Work out the finished part from the listing and answer in its coordinate system (mm). Face numbers are marked on the shaded views. A direction names the side the tool comes from. Coordinates: 2 decimals unless noted, no trailing zeros. Order: outer loops, then holes, each group sorted by start corner. A loop starts at its lowest first (then second) coordinate and runs counter-clockwise, first axis right, second up. Notation, with made-up numbers: M 8.25,31.5 L 35.25,31.5 A12 cw 35.25,41.5 Z; hole C -20,65.5 d6. An arc over 180 degrees is marked long. Answer in a Markdown table with one row per item. Add a question column.
Item 1: Which of the six approach directions +Z, -Z, +X, -X, +Y, -Y give full straight-line access (tool end or side, diameter ignored) to the marked faces 1 and 2?
Item 2: Flat-ended cylindrical pins translate along their axes: pin 1 Ø0.9 at (x, z) = (-1, 0.5) entering from -Y; pin 2 Ø0.9 at (x, y) = (-1.5, 0.5) entering from -Z; pin 3 Ø0.7 at (x, z) = (-1, 0) entering from +Y. Find the tip coordinate at first contact, or state that the pin passes through.
Item 3: The mould has two halves that part along Y. Classify the marked faces 3, 4 and 5: released by +Y, released by -Y, zero draft, split by the parting line, or undercut.
Item 4: The part is cut by section B-B (z = 0). Write down the section's boundary in (x, y).
Item 5: Consider line 1 (X direction, y = -0.65, z = 0.2); line 2 (Y direction, x = -1, z = -1.1); line 3 (X direction, y = 0.4, z = -1.45). Determine where each line is inside the solid, lowest interval first. Write a range as from..to.
Item 6: The part is cut by section A-A (x = 7.5). Write down the section's boundary in (y, z).
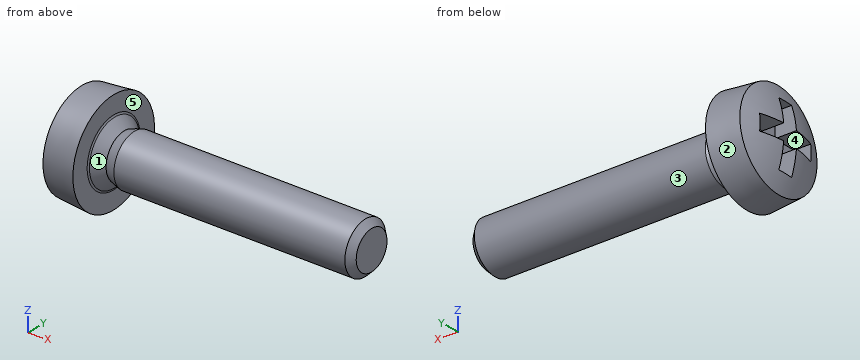
from build123d import *

# Parameters (mm, degrees)
SKETCH2_R               = 1.257053568
BOSS_EXTRUDE1_DEPTH     = 0.4
BOSS_EXTRUDE1_TAPER     = 43.516406292
SKETCH3_R               = 0.87725
BOSS_EXTRUDE2_DEPTH     = 0.4
BOSS_EXTRUDE2_DRAFT     = -17.059940879
SKETCH4_R               = 1
BOSS_EXTRUDE3_DEPTH     = 9.2
CUT_EXTRUDE1_REACH      = 13.222
CUT_EXTRUDE1_END_RADIUS = 4
CHAMFER1_SIZE           = 0.2455
FILLET1_R               = 0.1


with BuildPart() as part:
    # Sketch1 → Revolve1 (revolve)
    with BuildSketch(Plane(origin=(0, 0, 0), x_dir=(-1, 0, 0), z_dir=(0, 0, -1)), mode=Mode.PRIVATE) as revolve1_sk:
        with BuildLine():
            Line((0, 2), (0, 0))
            Line((0, 0), (1.72, 0))
            ThreePointArc((1.72, 0), (1.599364053, 0.974953612), (1.244732728, 1.891099997))
            Line((1.244732728, 1.891099997), (0, 2))
        make_face()
    revolve(revolve1_sk.sketch.rotate(Axis((0, 0, 0), (-1, 0, 0)), 270), axis=Axis((0, 0, 0), (-1, 0, 0)))

    # Sketch2 → Boss-Extrude1 (add)
    with BuildSketch(Plane(origin=(0, 0, 0), x_dir=(0, 0, -1), z_dir=(1, 0, 0))):
        Circle(SKETCH2_R)
    extrude(amount=BOSS_EXTRUDE1_DEPTH, taper=BOSS_EXTRUDE1_TAPER)


with BuildPart() as boss_extrude2_tool:
    # Sketch3 → Boss-Extrude2 (with draft: the straight prism first)
    with BuildSketch(Plane(origin=(0.4, 0, 0), x_dir=(0, 0, -1), z_dir=(1, 0, 0))):
        Circle(SKETCH3_R)
    extrude(amount=BOSS_EXTRUDE2_DEPTH)
    # Boss-Extrude2: the draft: its side faces are tilted about the plane it starts from
    boss_extrude2_sides = [boss_extrude2_tool.faces().sort_by_distance(p)[0] for p in [
        (0.6, 0, 0.87725),
    ]]
    draft(boss_extrude2_sides, Plane(origin=(0.4, 0, 0), x_dir=(0, 0, -1), z_dir=(1, 0, 0)), BOSS_EXTRUDE2_DRAFT)


with BuildPart() as part_1:
    add(part.part)

    # Boss-Extrude2: add boss_extrude2_tool
    add(boss_extrude2_tool.part)

    # Sketch4 → Boss-Extrude3 (add)
    with BuildSketch(Plane(origin=(0.8, 0, 0), x_dir=(0, 0, -1), z_dir=(1, 0, 0))):
        Circle(SKETCH4_R)
    extrude(amount=BOSS_EXTRUDE3_DEPTH)

    # Cut-Extrude1: up to this sphere (the profile starts inside it)
    cut_extrude1_end = Location((2.28, 0, 0)) * Sphere(CUT_EXTRUDE1_END_RADIUS, mode=Mode.PRIVATE)
    # Sketch5 → Cut-Extrude1 (cut, up to the surface)
    with BuildSketch(Plane(origin=(-0.86, 0, 0), x_dir=(0, 0, -1), z_dir=(1, 0, 0)), mode=Mode.PRIVATE) as cut_extrude1_sk1:
        Polygon((0.3125, 0.3125), (0.3125, 1.25), (-0.3125, 1.25), (-0.3125, 0.3125), (-1.25, 0.3125), (-1.25, -0.3125), (-0.3125, -0.3125), (-0.3125, -1.25), (0.3125, -1.25), (0.3125, -0.3125), (1.25, -0.3125), (1.25, 0.3125), align=None)
    cut_extrude1_tool1 = extrude(cut_extrude1_sk1.sketch, amount=-CUT_EXTRUDE1_REACH, mode=Mode.PRIVATE) & cut_extrude1_end
    add(cut_extrude1_tool1.solids().sort_by_distance((-0.86, 0, 0))[0], mode=Mode.SUBTRACT)

    # Chamfer1
    chamfer1_edges = [part_1.edges().sort_by_distance(p)[0] for p in [
        (10, 0, 1),
    ]]
    chamfer(chamfer1_edges, length=CHAMFER1_SIZE)

    # Fillet1
    fillet1_edges = [part_1.edges().sort_by_distance(p)[0] for p in [
        (0, 0, 1.257053568),
    ]]
    fillet(fillet1_edges, radius=FILLET1_R)


solid = part_1.part
Reply:
| question | item | result |
|---|---|---|
| 1 | face 1 | none |
| 1 | face 2 | -X |
| 2 | pin 1 | stops at y = -1.93 |
| 2 | pin 2 | stops at z = -1.89 |
| 2 | pin 3 | stops at y = 1.94 |
| 3 | face 3 | split by the parting line |
| 3 | face 4 | undercut |
| 3 | face 5 | zero draft |
| 4 | outline | M -1.52,-1.25 A4 ccw -1.24,-1.89 L 0,-2 L 0,-1.3 A0.1 cw 0.03,-1.23 L 0.4,-0.88 L 0.8,-1 L 9.75,-1 L 10,-0.75 L 10,0.75 L 9.75,1 L 0.8,1 L 0.4,0.88 L 0.03,1.23 A0.1 cw 0,1.3 L 0,2 L -1.24,1.89 A4 ccw -1.52,1.25 L -0.86,1.25 L -0.86,-1.25 Z |
| 5 | line 1 | x = -0.86..10 |
| 5 | line 2 | y = -1.56..-0.31, 0.31..1.56 |
| 5 | line 3 | x = -1.43..0 |
| 6 | outline | C 0,0 d2 |
